from build123d import *

# Parameters (mm, degrees)
SKIZZE1_W                       = 25
SKIZZE1_H                       = 10
SKIZZE1_R                       = 1.65
AUFSATZ_LINEAR_AUSTRAGEN1_DEPTH = 2.5
SKIZZE2_W                       = 15
SKIZZE2_H                       = 2.5
AUFSATZ_LINEAR_AUSTRAGEN2_DEPTH = 8.5
VERRUNDUNG1_R                   = 2
SKIZZE3_R                       = 3.2
SCHNITT_LINEAR_AUSTRAGEN1_DEPTH = 8.5


with BuildPart() as part:
    # Skizze1 → Aufsatz-Linear austragen1 (new body)
    with BuildSketch(Plane.XY):
        with Locations((12.5, 5)):
            Rectangle(SKIZZE1_W, SKIZZE1_H)
        with Locations((20, 5)):
            Circle(SKIZZE1_R, mode=Mode.SUBTRACT)
    extrude(amount=AUFSATZ_LINEAR_AUSTRAGEN1_DEPTH)

    # Skizze2 → Aufsatz-Linear austragen2 (add)
    with BuildSketch(Plane.XY.offset(2.5)):
        with Locations((7.5, 8.75)):
            Rectangle(SKIZZE2_W, SKIZZE2_H)
    extrude(amount=AUFSATZ_LINEAR_AUSTRAGEN2_DEPTH)

    # Verrundung1
    verrundung1_edges = [part.edges().sort_by_distance(p)[0] for p in [
        (15, 8.75, 2.5),
        (0, 8.75, 11),
        (15, 8.75, 11),
    ]]
    fillet(verrundung1_edges, radius=VERRUNDUNG1_R)

    # Skizze3 → Schnitt-Linear austragen1 (cut)
    with BuildSketch(Plane.XZ.offset(-7.5)):
        with Locations(Location((7.5, 6.6, 0), (0, 0, 270))):
            Circle(SKIZZE3_R)
    extrude(amount=-SCHNITT_LINEAR_AUSTRAGEN1_DEPTH, mode=Mode.SUBTRACT)


solid = part.part
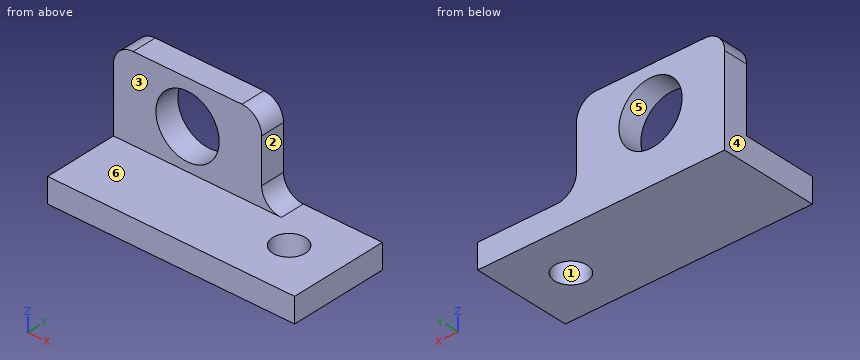
The model under review builds one solid part; all positions refer to its coordinate system, in mm. Face numbers are marked on the shaded views. A direction names the side the tool comes from. Round coordinates to 2 decimals unless told otherwise and drop trailing zeros. Order: outer loops, then holes, each group sorted by start corner. A loop starts at its lowest first (then second) coordinate and runs counter-clockwise, first axis right, second up. Notation, with made-up numbers: (-33.75, 82.25) -> (25.25, 82.25) arc R16 cw to (25.25, 100.25) -> close; hole circle Ø9 at (74, 57.25). An arc over 180 degrees is marked (long way). Return JSON: item names as keys, results as strings.
1. Take a section at B-B (x = 20). Write out the cut boundary in (y, z), then the cut area to 4 significant figures.
Answer block:
{"outline": "(0, 0) -> (3.35, 0) -> (3.35, 2.5) -> (0, 2.5) -> close; (6.65, 0) -> (10, 0) -> (10, 2.5) -> (6.65, 2.5) -> close", "area": "16.75 mm²"}
2. For the marked faces 1, 2 and 3, list the 3-axis set-ups (+Z, -Z, +X, -X, +Y, -Y) from which the entire face can be reached by the end or side of a thin tool; tool diameter is ignored.
Answer block:
{"face 1": "+Z, -Z", "face 2": "+Z, +X, +Y, -Y", "face 3": "+Z, +X, -X, -Y"}
3. For L1, parallel to X at y = 9.3, z = 6.6; L2, parallel to Y at x = 20, z = 1.55; L3, parallel to Y at x = 12.5, z = 9.5, list the stretches that pass through material, from the lowest coordinate up. Write a range as [from, to].
Answer block:
{"L1": "x = [0, 4.3], [10.7, 15]", "L2": "y = [0, 3.35], [6.65, 10]", "L3": "y = [7.5, 10]"}
4. Take a section at C-C (z = 1). Write out the cut boundary in (x, y).
Answer block:
{"outline": "(0, 0) -> (25, 0) -> (25, 10) -> (0, 10) -> close; hole circle Ø3.3 at (20, 5)"}
5. Take a section at A-A (y = 5). Write out the cut boundary in (x, z), then the cut area to 4 significant figures.
Answer block:
{"outline": "(0, 0) -> (18.35, 0) -> (18.35, 2.5) -> (0, 2.5) -> close; (21.65, 0) -> (25, 0) -> (25, 2.5) -> (21.65, 2.5) -> close", "area": "54.25 mm²"}
6. Insertion check: P1, Ø4.5, axis at x = 20, y = 5, coming from the +Z side; P2, Ø0.8, axis at y = 8.5, z = 6, coming from the +X side; P3, Ø6, axis at x = 11, z = 7, coming from the -Y side. Each pin has a flat end and moves straight along its axis. Give the tip position at first contact, or say it passes through.
Answer block:
{"P1": "stops at z = 2.5", "P2": "stops at x = 15", "P3": "stops at y = 7.5"}
7. Take a section at D-D (y = 8.5). Write out the cut boundary in (x, z).
Answer block:
{"outline": "(0, 0) -> (25, 0) -> (25, 2.5) -> (17, 2.5) arc R2 cw to (15, 4.5) -> (15, 9) arc R2 ccw to (13, 11) -> (2, 11) arc R2 ccw to (0, 9) -> close; hole circle Ø6.4 at (7.5, 6.6)"}
8. The part is to be moulded in two halves that separate along Z. For the marked faces 4, 5 and 6, say which applies: +Z half, -Z half, draft (parallel to the pull), parting line (faces both ways), or undercut.
Answer block:
{"face 4": "draft", "face 5": "undercut", "face 6": "+Z half"}
